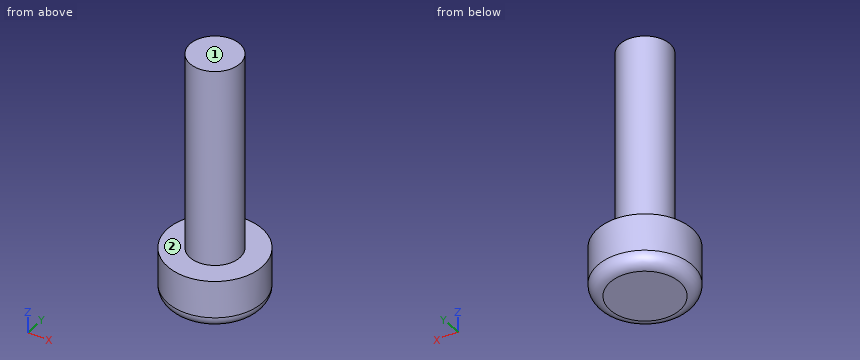
from build123d import *

# Parameters (mm, degrees)
SKETCH_2_R      = 1.9
EXTRUDE_1_DEPTH = 2
SKETCH_3_R      = 1
EXTRUDE_2_DEPTH = 8
FILLET_1_R      = 0.5


with BuildPart() as part:
    # ｽｹｯﾁ2 → ﾎﾞｽ - 押し出し1 (new body)
    with BuildSketch(Plane.XY):
        Circle(SKETCH_2_R)
    extrude(amount=EXTRUDE_1_DEPTH)

    # ｽｹｯﾁ3 → ﾎﾞｽ - 押し出し2 (add)
    with BuildSketch(Plane.XY.offset(2)):
        Circle(SKETCH_3_R)
    extrude(amount=EXTRUDE_2_DEPTH)

    # ﾌｨﾚｯﾄ1
    fillet_1_edges = [part.edges().sort_by_distance(p)[0] for p in [
        (-1.9, 0, 0),
    ]]
    fillet(fillet_1_edges, radius=FILLET_1_R)


solid = part.part
Could you check a few things on this model? Use its own coordinates, in mm. Face numbers are marked on the shaded views. A direction names the side the tool comes from. Give positions to 0.01 mm unless a question says otherwise; leave off trailing zeros. Order: outer loops, then holes, each group sorted by start corner. A loop starts at its lowest first (then second) coordinate and runs counter-clockwise, first axis right, second up. Notation, with made-up numbers: (84, 59) -> (100, 59) arc R7 cw to (100, 67) -> close; hole circle Ø2 at (55, 68). An arc over 180 degrees is marked (long way). Answer in a Markdown table with one row per item. Add a question column.
Item 1: Please list where these lines run through material, in increasing order: probe 1 along Z at (x, y) = (0.5, -1.2); probe 2 along X at (y, z) = (-0.7, 3.25); probe 3 along X at (y, z) = (-0.1, 5).
Item 2: Imagine slicing it at C-C (z = 7.75). List the corners of the cut face in (x, y) for me.
Item 3: Imagine slicing it at A-A (y = 0). List the corners of the cut face in (x, z) for me.
Item 4: Imagine slicing it at D-D (z = 1.25). List the corners of the cut face in (x, y) for me, and give its area (3 significant figures).
Item 5: For the marked faces 1 and 2, which set-ups out of +Z, -Z, +X, -X, +Y, -Y let a thin tool reach every point of the face, with its end or its side?
Item 6: I'm going to push flat-ended pins straight in: P1, Ø1, axis at x = 0.5, z = 7, coming from the +Y side; P2, Ø1.5, axis at x = -1.5, z = 6.5, coming from the +Y side; P3, Ø2, axis at x = -0.5, z = 6.5, coming from the -Y side. Where does each tip first touch, or does it pass through?
Result:
| question | item | result |
|---|---|---|
| 1 | probe 1 | 0 to 2 |
| 1 | probe 2 | -0.71 to 0.71 |
| 1 | probe 3 | -0.99 to 0.99 |
| 2 | outline | circle Ø2 at (0, 0) |
| 3 | outline | (-1.9, 0.5) arc R0.5 ccw to (-1.4, 0) -> (1.4, 0) arc R0.5 ccw to (1.9, 0.5) -> (1.9, 2) -> (1, 2) -> (1, 10) -> (-1, 10) -> (-1, 2) -> (-1.9, 2) -> close |
| 4 | outline | circle Ø3.8 at (0, 0) |
| 4 | area | 11.3 mm2 |
| 5 | face 1 | +Z, +X, -X, +Y, -Y |
| 5 | face 2 | +Z |
| 6 | P1 | y = 1 |
| 6 | P2 | y = 0.66 |
| 6 | P3 | y = -1 |
